from build123d import *

# Parameters (mm, degrees)
SKETCH1_R           = 5
BOSS_EXTRUDE1_DEPTH = 220
SKETCH4_R           = 3.2
BOSS_EXTRUDE3_DEPTH = 6
BOSS_EXTRUDE4_DEPTH = 220
SKETCH5_R           = 1.37
CUT_EXTRUDE1_DEPTH  = 7
SKETCH6_R           = 1.37
CUT_EXTRUDE2_DEPTH  = 7


with BuildPart() as part:
    # Sketch1 → Boss-Extrude1 (new body)
    with BuildSketch(Plane.XY):
        Circle(SKETCH1_R)
        with BuildLine():
            Line((-4, -3), (-7, -8.196152423))
            Line((-7, -8.196152423), (7, -8.196152423))
            Line((7, -8.196152423), (4, -3))
            ThreePointArc((4, -3), (0, 5), (-4, -3))
        make_face()
        with BuildLine():
            Line((28.8, -3), (31.8, -8.196152423))
            Line((31.8, -8.196152423), (17.8, -8.196152423))
            Line((17.8, -8.196152423), (20.8, -3))
            ThreePointArc((20.8, -3), (24.8, 5), (28.8, -3))
        make_face()
    extrude(amount=BOSS_EXTRUDE1_DEPTH)

    # Sketch4 → Boss-Extrude3 (add)
    with BuildSketch(Plane.XZ.offset(8.196152423)):
        with Locations((0, 196.8)):
            Circle(SKETCH4_R)
        with Locations((24.8, 196.8)):
            Circle(SKETCH4_R)
        with Locations((24.8, 172)):
            Circle(SKETCH4_R)
        with Locations((24.8, 147.2)):
            Circle(SKETCH4_R)
        with Locations((24.8, 122.4)):
            Circle(SKETCH4_R)
        with Locations((24.8, 97.6)):
            Circle(SKETCH4_R)
        with Locations((24.8, 72.8)):
            Circle(SKETCH4_R)
        with Locations((24.8, 48)):
            Circle(SKETCH4_R)
        with Locations((24.8, 23.2)):
            Circle(SKETCH4_R)
        with Locations((0, 172)):
            Circle(SKETCH4_R)
        with Locations((0, 147.2)):
            Circle(SKETCH4_R)
        with Locations((0, 122.4)):
            Circle(SKETCH4_R)
        with Locations((0, 97.6)):
            Circle(SKETCH4_R)
        with Locations((0, 72.8)):
            Circle(SKETCH4_R)
        with Locations((0, 48)):
            Circle(SKETCH4_R)
        with Locations((0, 23.2)):
            Circle(SKETCH4_R)
    extrude(amount=BOSS_EXTRUDE3_DEPTH)

    # Sketch3 → Boss-Extrude4 (add)
    with BuildSketch(Plane.XY.offset(220)):
        Polygon((7, -8.196152423), (17.8, -8.196152423), (18.65, -8.196152423), (18.65, -6.723909236), (6.15, -6.723909236), (6.15, -8.196152423), align=None)
    extrude(amount=-BOSS_EXTRUDE4_DEPTH)

    # Sketch5 → Cut-Extrude1 (cut)
    with BuildSketch(Plane(origin=(0, 0, 0), x_dir=(-1, 0, 0), z_dir=(0, 0, -1))):
        Circle(SKETCH5_R)
        with Locations((-24.8, 0)):
            Circle(SKETCH5_R)
    extrude(amount=-CUT_EXTRUDE1_DEPTH, mode=Mode.SUBTRACT)

    # Sketch6 → Cut-Extrude2 (cut)
    with BuildSketch(Plane.XY.offset(220)):
        Circle(SKETCH6_R)
        with Locations((24.8, 0)):
            Circle(SKETCH6_R)
    extrude(amount=-CUT_EXTRUDE2_DEPTH, mode=Mode.SUBTRACT)


solid = part.part
CAD build for the part. Positions are in the model's coordinates, mm. A direction names the side the tool comes from. Round coordinates to 2 decimals unless told otherwise and drop trailing zeros. Write each loop counter-clockwise with the first axis right and the second up, starting at its lowest first coordinate (ties: lowest second). Pieces come first, ordered by that corner, then holes. Notation, with made-up numbers: M 77.5,19.5 L 118.5,19.5 A23 cw 118.5,46.5 Z; hole C -34,-12 d3. An arc over 180 degrees is marked long. Use a Markdown table: item, result. Add a question column.
1. Drill centre lines: probe 1 along X at (y, z) = (-11.75, 97.5); probe 2 along Y at (x, z) = (24.8, 216.75); probe 3 along Y at (x, z) = (18.5, 100). Where is each one in solid material? Low to high.
2. Flat gauge pins, fed straight in: P1, Ø5, axis at x = 15.5, z = 153.5, coming from the +Y side; P2, Ø1.5, axis at x = 16.5, z = 71, coming from the -Y side; P3, Ø2, axis at x = 24.5, y = -0.5, coming from the -Z side; P4, Ø1.5, axis at y = -1.5, z = 96, coming from the +X side. Where does each tip first touch, or does it go through?
3. Slice it at A-A on z = 122.4. Give the cut face in (x, y), then the cut area to 3 significant figures.
4. 3-axis set-ups, long thin cutter, end or side, ignore diameter. For faces 1 (the face through (27.852, -11.154, 24.161)), 2 (the face through (19.71, -4.89, 108.46)), 3 (the face through (30.3, -5.6, 108.5)): which of +Z, -Z, +X, -X, +Y, -Y reach the whole face in a straight line?
5. Pull direction Y, two halves, no side cores. Call faces 4 (the face through (-0.417, -11.154, 175.173)), 5 (the face through (5.09, -4.89, 108.46)), 6 (the face through (25, -14.196, 147)): released by +Y, released by -Y, zero draft, split by the parting line, or undercut.
Reply:
| question | item | result |
|---|---|---|
| 1 | probe 1 | x = -3.2 to 3.2, 21.6 to 28 |
| 1 | probe 2 | y = -8.2 to -1.37, 1.37 to 5 |
| 1 | probe 3 | y = -8.2 to -6.72 |
| 2 | P1 | stops at y = -6.72 |
| 2 | P2 | stops at y = -8.2 |
| 2 | P3 | stops at z = 0 |
| 2 | P4 | stops at x = 29.74 |
| 3 | outline | M -7,-8.2 L -3.2,-8.2 L -3.2,-14.2 L 3.2,-14.2 L 3.2,-8.2 L 21.6,-8.2 L 21.6,-14.2 L 28,-14.2 L 28,-8.2 L 31.8,-8.2 L 28.8,-3 A5 ccw long 20.8,-3 L 18.65,-6.72 L 6.15,-6.72 L 4,-3 A5 ccw long -4,-3 Z |
| 3 | area | 343 mm^2 |
| 4 | face 1 | -Y |
| 4 | face 2 | +Z, -Z |
| 4 | face 3 | +Z, -Z, +X |
| 5 | face 4 | zero draft |
| 5 | face 5 | undercut |
| 5 | face 6 | released by -Y |
